Could you check a few things on this model? Use its own coordinates, in mm. A direction names the side the tool comes from. Coordinates: 2 decimals unless noted, no trailing zeros. Order: outer loops, then holes, each group sorted by start corner. A loop starts at its lowest first (then second) coordinate and runs counter-clockwise, first axis right, second up. Notation, with made-up numbers: (62, -36.75) - (118, -36.75) arc R12 ccw to (118, -31.75) - close; hole circle Ø8 at (5.5, 50). An arc over 180 degrees is marked (long way). Answer as a JSON object with one key per item and string values. Group by question number.
(1) Will these pins go through, and if not, where does the flat tip stop? P1, Ø1.9, axis at x = -24.11, z = 40.13, coming from the -Y side; P2, Ø2.5, axis at y = -10.5, z = 21.5, coming from the -X side; P3, Ø2.5, axis at y = -10, z = 23, coming from the +X side; P4, Ø10, axis at x = -13.5, z = 21, coming from the +Y side.
(2) Which directions (+Z, -Z, +X, -X, +Y, -Y) give clear straight access to the entire face, cutting with the end or side of a thin tool? Please do faces 4 (the cylindrical face through (-23.51, 1.97, 40.05)), 5 (the cylindrical face through (-24.018, -10.846, 27.625)), 6 (the flat face through (-19.107, -10, 23)), 7 (the cylindrical face through (-16.38, -2.11, 23.55)), 8 (the flat face through (-24, 2, 47.625)).
(3) Please list where these lines run through material, in increasing order: probe 1 along Y at (x, z) = (-16, 26); probe 2 along X at (y, z) = (-1.25, 21.25); probe 3 along Y at (x, z) = (-21, 30.75).
(4) Imagine slicing it at B-B, the plane y = -20.5. Write out the boundary of the cut face in (x, z), and give its area (3 significant figures).
(5) Imagine slicing it at A-A, the plane x = -37. Write out the boundary of the cut face in (y, z), and give its area (3 significant figures).
(6) Imagine slicing it at C-C, the plane y = -4. Write out the boundary of the cut face in (x, z).
(7) We'd pull the mould along X, two halves only. Please class faces 1 (the flat face through (-43.107, 1, 25)), 2 (the flat face through (-17, -8.4, 23)), 3 (the flat face through (-24, 4, 32)): pulls with the +X half, pulls with the -X half, needs draft (parallel to the pull), parting line crosses it, or undercut.
(8) Imagine slicing it at D-D, the plane x = -25.5. Write out the boundary of the cut face in (y, z), and give its area (3 significant figures).
from build123d import *

# Parameters (mm, degrees)
CROQUIS2_R              = 0.6
SALIENTE_EXTRUIR1_DEPTH = 4
SALIENTE_EXTRUIR2_DEPTH = 22
REDONDEO1_R             = 10
REDONDEO2_R             = 10
CROQUIS4_R              = 2
CORTAR_EXTRUIR1_DEPTH   = 15.4
CROQUIS5_W              = 9
CROQUIS5_H              = 3
CORTAR_EXTRUIR2_DEPTH   = 12


with BuildPart() as part:
    # Croquis2 → Saliente-Extruir1 (new body)
    with BuildSketch(Plane(origin=(0, 0, 0), x_dir=(1, 0, 0), z_dir=(0, 1, 0))):
        with BuildLine():
            Line((-43.107082341, -17.625158928), (-5.107082341, -17.625158928))
            Line((-5.107082341, -17.625158928), (-5.107082341, -37.625158928))
            ThreePointArc((-5.107082341, -37.625158928), (-8.036014529, -44.69622674), (-15.107082341, -47.625158928))
            Line((-15.107082341, -47.625158928), (-33.107082341, -47.625158928))
            ThreePointArc((-33.107082341, -47.625158928), (-40.178150153, -44.69622674), (-43.107082341, -37.625158928))
            Line((-43.107082341, -37.625158928), (-43.107082341, -17.625158928))
        make_face()
        with Locations(Location((-24.107082341, -40.125158928, 0), (0, 0, 270))):
            Circle(CROQUIS2_R, mode=Mode.SUBTRACT)
    extrude(amount=SALIENTE_EXTRUIR1_DEPTH)

    # Croquis3 → Saliente-Extruir2 (add)
    with BuildSketch(Plane.XZ):
        with BuildLine():
            Line((-43.107082341, 17.625158928), (-5.107082341, 17.625158928))
            Line((-5.107082341, 17.625158928), (-5.107082341, 37.625158928))
            ThreePointArc((-5.107082341, 37.625158928), (-24.107082341, 27.625158928), (-43.107082341, 37.625158928))
            Line((-43.107082341, 37.625158928), (-43.107082341, 17.625158928))
        make_face()
    extrude(amount=SALIENTE_EXTRUIR2_DEPTH)

    # Redondeo1
    redondeo1_edges = [part.edges().sort_by_distance(p)[0] for p in [
        (-43.107082341, -11, 37.625158928),
    ]]
    fillet(redondeo1_edges, radius=REDONDEO1_R)

    # Redondeo2
    redondeo2_edges = [part.edges().sort_by_distance(p)[0] for p in [
        (-5.107082341, -11, 37.625158928),
    ]]
    fillet(redondeo2_edges, radius=REDONDEO2_R)

    # Croquis4 → Cortar-Extruir1 (cut)
    with BuildSketch(Plane(origin=(0, 4, 0), x_dir=(1, 0, 0), z_dir=(0, 1, 0))):
        with Locations(Location((-33.607082341, -22.625158928, 0), (0, 0, 270))):
            Circle(CROQUIS4_R)
        with Locations(Location((-14.607082341, -22.625158928, 0), (0, 0, 270))):
            Circle(CROQUIS4_R)
    extrude(amount=-CORTAR_EXTRUIR1_DEPTH, mode=Mode.SUBTRACT)

    # Croquis5 → Cortar-Extruir2 (cut)
    with BuildSketch(Plane(origin=(0, 0, 17.625158928), x_dir=(-1, 0, 0), z_dir=(0, 0, -1))):
        with Locations((33.607082341, -9.9)):
            Rectangle(CROQUIS5_W, CROQUIS5_H)
        with Locations((14.607082341, -9.9)):
            Rectangle(CROQUIS5_W, CROQUIS5_H)
    extrude(amount=-CORTAR_EXTRUIR2_DEPTH, mode=Mode.SUBTRACT)


solid = part.part
Result set:
{
 "1": {"P1": "stops at y = 0", "P2": "stops at x = -43.01", "P3": "stops at x = -5.53", "P4": "stops at y = 4"},
 "2": {"face 4": "+Y, -Y", "face 5": "+Z, -Y", "face 6": "+Z, -Z", "face 7": "+Y", "face 8": "+Z, +X, -X, +Y, -Y"},
 "3": {"probe 1": "y = -22 to -11.4, -8.4 to 4", "probe 2": "x = -42.82 to -35.06, -32.15 to -16.06, -13.15 to -5.39", "probe 3": "y = 0 to 4"},
 "4": {"outline": "(-43.11, 17.63) - (-5.11, 17.63) - (-5.11, 18.87) arc R10 ccw to (-17.83, 28.5) arc R23.05 cw to (-30.38, 28.5) arc R10 ccw to (-43.11, 18.87) - close", "area": "372 mm^2"},
 "5": {"outline": "(-22, 17.63) - (-11.4, 17.63) - (-11.4, 28.09) - (-22, 28.09) - close; (-8.4, 17.63) - (4, 17.63) - (4, 46.84) - (0, 46.84) - (0, 28.09) - (-8.4, 28.09) - close", "area": "316 mm^2"},
 "6": {"outline": "(-43.11, 17.63) - (-5.11, 17.63) - (-5.11, 18.87) arc R10 ccw to (-17.83, 28.5) arc R23.05 cw to (-30.38, 28.5) arc R10 ccw to (-43.11, 18.87) - close; hole circle Ø4 at (-33.61, 22.63); hole circle Ø4 at (-14.61, 22.63)"},
 "7": {"face 1": "pulls with the -X half", "face 2": "undercut", "face 3": "needs draft"},
 "8": {"outline": "(-22, 17.63) - (4, 17.63) - (4, 47.63) - (0, 47.63) - (0, 27.67) - (-22, 27.67) - close", "area": "341 mm^2"}
}
